```python
from build123d import *

# Parameters (mm, degrees)
F0_W     = 563
F0_H     = 243
F1_DEPTH = 35
F2_T     = -1.5
F5_R     = 4


with BuildPart() as f1:
    # F0 (on Top) → F1 (new body)
    with BuildSketch(Plane.XY):
        with Locations((184.3085842729, 121.5)):
            Rectangle(F0_W, F0_H)
    extrude(amount=-F1_DEPTH)

    # F2
    f2_openings = [f1.faces().sort_by_distance(p)[0] for p in [
        (184.308584, 121.5, -35),
    ]]
    offset(amount=F2_T, openings=f2_openings)

    # F6: sweep along a path in F4
    with BuildLine(Plane.XZ.offset(-121.5)) as f6_path:
        Line((114.3085842729, 0), (114.3085842729, 30))
        ThreePointArc((114.3085842729, 30), (117.237516461, 37.0710678119), (124.3085842729, 40))
        Line((124.3085842729, 40), (244.3085842729, 40))
        ThreePointArc((244.3085842729, 40), (251.3796520847, 37.0710678119), (254.3085842729, 30))
        Line((254.3085842729, 30), (254.3085842729, 0))
    # F5 (on face) → F6 (sweep)
    with BuildSketch(Plane.XY):
        with Locations((115.6852245331, 120.5054670572)):
            Circle(F5_R)
    sweep(path=f6_path.line)


solid = f1.part
```
Can you work these out from the model? Positions are in its coordinate system, mm. A direction names the side the tool comes from. Round coordinates to 2 decimals unless told otherwise and drop trailing zeros. Loops run counter-clockwise (first coordinate to the right, second up) from the corner with the lowest first, then second, coordinate; pieces in that order, holes last. Notation, with made-up numbers: M 51.25,19 L 87.25,19 A18 ccw 87.25,40 Z; hole C -20.75,26.25 d6. An arc over 180 degrees is marked long. Answer in a Markdown table with one row per item.
1. If we section it at D-D, the plane x = 357.5: Please give me the cut outline in (y, z).
Established:
| item | result |
|---|---|
| outline | M 0,-35 L 1.5,-35 L 1.5,-1.5 L 241.5,-1.5 L 241.5,-35 L 243,-35 L 243,0 L 0,0 Z |
2. On a 3-axis mill with a long thin cutter (end or side, diameter ignored), from which of +Z, -Z, +X, -X, +Y, -Y can I reach the whole of each face in a straight line? I mean faces 1 (the face through (180, 0, -17)), 2 (the face through (180, 1.5, -18)). Say none if no direction works.
Established:
| item | result |
|---|---|
| face 1 | +Z, -Z, +X, -X, -Y |
| face 2 | -Z |
3. Please list where these lines run through material, in increasing order: line 1 (X direction, y = 25, z = -24); line 2 (Y direction, x = 326.5, z = -2); line 3 (Z direction, x = 195.5, y = 233). Write a range as from..to.
Established:
| item | result |
|---|---|
| line 1 | -97.19..-95.69, 464.31..465.81 |
| line 2 | 0..1.5, 241.5..243 |
| line 3 | -1.5..0 |
4. If we section it at B-B, the plane y = 91: Please give me the cut outline in (x, z).
Established:
| item | result |
|---|---|
| outline | M -97.19,-35 L -95.69,-35 L -95.69,-1.5 L 464.31,-1.5 L 464.31,-35 L 465.81,-35 L 465.81,0 L -97.19,0 Z |
5. I'm going to push flat-ended pins straight in: pin 1 Ø12 at (x, y) = (253.5, 36) entering from -Z; pin 2 Ø8 at (x, y) = (288, 30.5) entering from +Z. Where does each tip first touch, or does it pass through?
Established:
| item | result |
|---|---|
| pin 1 | z = -1.5 |
| pin 2 | z = 0 |
6. If we section it at C-C, the plane x = 183: Please give me the cut outline in (y, z), plus the area to 3 significant figures.
Established:
| item | result |
|---|---|
| outline | M 0,-35 L 1.5,-35 L 1.5,-1.5 L 241.5,-1.5 L 241.5,-35 L 243,-35 L 243,0 L 0,0 Z; C 120.51,38.62 d8 |
| area | 515 mm² |
7. Thinking about a two-plate mould opening in X: for faces 3 (the face through (180, 243, -17)), 4 (the face through (-97.191, 120, -17)), 5 (the face through (180, 123, -1.5)), 6 (the face through (465.809, 120, -17)), which applies, pulls with the +X half, pulls with the -X half, needs draft (parallel to the pull), parting line crosses it, or undercut?
Established:
| item | result |
|---|---|
| face 3 | needs draft |
| face 4 | pulls with the -X half |
| face 5 | undercut |
| face 6 | pulls with the +X half |
8. If we section it at A-A, the plane z = -17.5: Please give me the cut outline in (x, y).
Established:
| item | result |
|---|---|
| outline | M -97.19,0 L 465.81,0 L 465.81,243 L -97.19,243 Z; hole M -95.69,1.5 L 464.31,1.5 L 464.31,241.5 L -95.69,241.5 Z |
